Design review of the part built by this model. Coordinates are the model's own, in mm. Round coordinates to 2 decimals unless told otherwise and drop trailing zeros. Loops run counter-clockwise (first coordinate to the right, second up) from the corner with the lowest first, then second, coordinate; pieces in that order, holes last. Notation, with made-up numbers: M 63.5,15.5 L 83.5,15.5 A17 cw 83.5,33.5 Z; hole C -15,-32.75 d7. An arc over 180 degrees is marked long. One line per item, written item: value. Start each with the question number.
Item 1: Clearance check with a flat-ended pin moving along its axis: pin 1 (3 mm diameter, centred on x = -1.5, y = 2, fed in from +Z). State where the tip first meets the part, or that it passes through.
Item 2: Mouldability with a two-part tool opening along Z and no side actions: class faces 1 (the flat face through (0, 4.7, 0)), 2 (the cylindrical face through (0, 2, 12)), 3 (the cylindrical face through (0.228, 2.465, 7.265)), 4 (the flat face through (0, 0, 0)) as released by +Z, released by -Z, zero draft, split by the parting line, or undercut.
Item 3: For line 1 along X through (y, z) = (1.8, 9); line 2 along Z through (x, y) = (0, 3.45); line 3 along Z through (x, y) = (-0.7, 3), list the stretches that pass through material, from the lowest coordinate up.
Item 4: We need section B-B (z = 8.75). Write out the cut boundary in (x, y).
Item 5: We need section D-D (x = -1.3). Write out the cut boundary in (y, z), then the cut area to 3 significant figures.
Item 6: We need section A-A (x = 0). Write out the cut boundary in (y, z), then the cut area to 3 significant figures.
Item 7: We need section C-C (y = 3.5). Write out the cut boundary in (x, z), then the cut area to 3 significant figures.
Autodesk Inventor part; units mm, degrees
ref_plane "YZ Plane" through (0, 0, 0) normal (1, 0, 0) x (0, 1, 0)
ref_plane "XZ Plane" through (0, 0, 0) normal (0, 1, 0) x (-1, 0, 0)
ref_plane "XY Plane" through (0, 0, 0) normal (0, 0, 1) x (1, 0, 0)
sketch "Sketch1" plane through (0, 0, 0) normal (0, 1, 0) x (-1, 0, 0)
  circle A0 centre (0, 9) radius 1.75
  circle A1 centre (0, -9) radius 1.75
  circle A2 centre (0, 9) radius 3
  circle A3 centre (0, -9) radius 3
  line L0 (3, 9) -> (-3, 9)
  line L1 (-3, 9) -> (-3, -9)
  line L2 (-3, -9) -> (3, -9)
  line L3 (3, -9) -> (3, 9)
  point P0 (0, 0)
  point P1 (-3, 9)
  point P2 (3, -9)
  dimension "d6" = 6
  dimension "d7" = 6
  dimension "d0" = 3.5
  dimension "d1" = 3.5
  dimension "d2" = 9
  dimension "d3" = 9
  dimension "d4" = 0
  dimension "d5" = 0
  dimension "d8" = 18
  dimension "d9" = 6
extrude "Extrusion1" add sketch "Sketch1" along normal blind 5 contours L0 A2 A0 | A0 L0 A2 | L3 A3 L1 A2 | L2 A1 A3 | A3 L2 A1
sketch "Sketch2" plane through (0, 5, 0) normal (0, 1, 0) x (1, 0, 0)
  line L0 (-3, 9) -> (-3, -9)
  line L1 (3, -9) -> (3, 9)
  line L2 (-3, -6) -> (3, -6)
  line L3 (3, -6) -> (3, 6)
  line L4 (3, 6) -> (-3, 6)
  line L5 (-3, 6) -> (-3, -6)
  point P0 (0, 0)
  point P1 (3, -6)
  dimension "d12" = 6
  dimension "d13" = 6
extrude "Extrusion2" cut sketch "Sketch2" against normal blind 0.3
properties part number "Belt Holder"
A:
1. pin 1: z = 12
2. face 1: undercut
2. face 2: released by +Z
2. face 3: undercut
2. face 4: zero draft
3. line 1: -3 to -1.75, 1.75 to 3
3. line 2: -12 to -10.75, -7.25 to 7.25, 10.75 to 12
3. line 3: -11.92 to -10.6, -7.4 to 7.4, 10.6 to 11.92
4. outline: M -3,0 L -1.73,0 L -1.73,5 L -3,5 Z; M 1.73,0 L 3,0 L 3,5 L 1.73,5 Z
5. outline: M 0,-11.7 L 5,-11.7 L 5,-10.17 L 0,-10.17 Z; M 0,-7.83 L 5,-7.83 L 5,-6 L 4.7,-6 L 4.7,6 L 5,6 L 5,7.83 L 0,7.83 Z; M 0,10.17 L 5,10.17 L 5,11.7 L 0,11.7 Z
5. area: 90.0 mm2
6. outline: M 0,-12 L 5,-12 L 5,-10.75 L 0,-10.75 Z; M 0,-7.25 L 5,-7.25 L 5,-6 L 4.7,-6 L 4.7,6 L 5,6 L 5,7.25 L 0,7.25 Z; M 0,10.75 L 5,10.75 L 5,12 L 0,12 Z
6. area: 81.4 mm2
7. outline: M -3,-9 A3 ccw 3,-9 L 3,9 A3 ccw -3,9 Z; hole C 0,-9 d3.5; hole C 0,9 d3.5
7. area: 117 mm2
